```python
from build123d import *

# Parameters (mm, degrees)
EXTRUDE1_DEPTH                               = 38.1
F_3_8_CLEARANCE_HOLE1_D                      = 10.31748
TAPPED_HOLE_FOR_1_4_20_HELICOIL3_D           = 6.7564
TAPPED_HOLE_FOR_1_4_20_HELICOIL3_DEPTH       = 22.86
TAPPED_HOLE_FOR_1_4_20_HELICOIL3_CBORE_D     = 8.09498
TAPPED_HOLE_FOR_1_4_20_HELICOIL3_CBORE_DEPTH = 15.748
TAPPED_HOLE_FOR_1_4_20_HELICOIL3_TIP         = 2.029827343
TAPPED_HOLE_FOR_1_4_20_HELICOIL1_D           = 6.7564
TAPPED_HOLE_FOR_1_4_20_HELICOIL1_CBORE_D     = 8.09498
TAPPED_HOLE_FOR_1_4_20_HELICOIL1_CBORE_DEPTH = 15.748
FILLET1_R                                    = 5.08
F_3_16_0_1875_DIAMETER_HOLE1_REACH           = 70.58
F_3_16_0_1875_DIAMETER_HOLE1_BORE_R          = 2.38125
CHAMFER1_SIZE                                = 2.54


with BuildPart() as part:
    # Sketch1 → Extrude1 (new body)
    with BuildSketch(Plane.XY):
        Polygon((-73.66, 49.53), (-73.66, 68.58), (0, 68.58), (0, 0), (-38.1, 0), (-38.1, 49.53), align=None)
    extrude(amount=EXTRUDE1_DEPTH)

    # 3/8 Clearance Hole1 (through all)
    with Locations(Plane(origin=(-59.69, 68.58, 19.05), x_dir=(0, 0, 1), z_dir=(0, 1, 0))):
        with Locations((0, 0)):
            Hole(F_3_8_CLEARANCE_HOLE1_D / 2)

    # Tapped Hole for 1/4-20 Helicoil3
    with Locations(Plane(origin=(0, 59.563, 19.05), x_dir=(0, 0, 1), z_dir=(1, 0, 0))):
        with Locations((0, 0)):
            CounterBoreHole(TAPPED_HOLE_FOR_1_4_20_HELICOIL3_D / 2, TAPPED_HOLE_FOR_1_4_20_HELICOIL3_CBORE_D / 2, TAPPED_HOLE_FOR_1_4_20_HELICOIL3_CBORE_DEPTH, depth=TAPPED_HOLE_FOR_1_4_20_HELICOIL3_DEPTH)
            with Locations((0, 0, -(TAPPED_HOLE_FOR_1_4_20_HELICOIL3_DEPTH + TAPPED_HOLE_FOR_1_4_20_HELICOIL3_TIP / 2))):  # 118° drill point
                Cone(0, TAPPED_HOLE_FOR_1_4_20_HELICOIL3_D / 2, TAPPED_HOLE_FOR_1_4_20_HELICOIL3_TIP, mode=Mode.SUBTRACT)

    # Tapped Hole for 1/4-20 Helicoil1 (through all)
    with Locations(Plane(origin=(0, 14.986, 19.05), x_dir=(0, 0, 1), z_dir=(1, 0, 0))):
        with Locations((0, 0)):
            CounterBoreHole(TAPPED_HOLE_FOR_1_4_20_HELICOIL1_D / 2, TAPPED_HOLE_FOR_1_4_20_HELICOIL1_CBORE_D / 2, TAPPED_HOLE_FOR_1_4_20_HELICOIL1_CBORE_DEPTH)

    # Fillet1
    fillet1_edges = [part.edges().sort_by_distance(p)[0] for p in [
        (-38.1, 49.53, 19.05),
    ]]
    fillet(fillet1_edges, radius=FILLET1_R)

    # 3/16 (0.1875) Diameter Hole1 bore (on position points) → 3/16 (0.1875) Diameter Hole1 (cut, up to next)
    with BuildSketch(Plane(origin=(-19.05, 68.58, 19.05), x_dir=(0, 0, 1), z_dir=(0, 1, 0)), mode=Mode.PRIVATE) as f_3_16_0_1875_diameter_hole1_sk1:
        Circle(F_3_16_0_1875_DIAMETER_HOLE1_BORE_R)
    f_3_16_0_1875_diameter_hole1_tool1 = extrude(f_3_16_0_1875_diameter_hole1_sk1.sketch, amount=-F_3_16_0_1875_DIAMETER_HOLE1_REACH, mode=Mode.PRIVATE) & part.part
    add(f_3_16_0_1875_diameter_hole1_tool1.solids().sort_by_distance((-19.05, 68.58, 19.05))[0], mode=Mode.SUBTRACT)

    # Chamfer1
    chamfer1_edges = [part.edges().sort_by_distance(p)[0] for p in [
        (0, 34.29, 38.1),
        (-36.83, 68.58, 38.1),
        (-73.66, 59.055, 38.1),
        (-73.66, 59.055, 0),
        (-36.83, 68.58, 0),
        (0, 34.29, 0),
    ]]
    chamfer(chamfer1_edges, length=CHAMFER1_SIZE)


solid = part.part
```
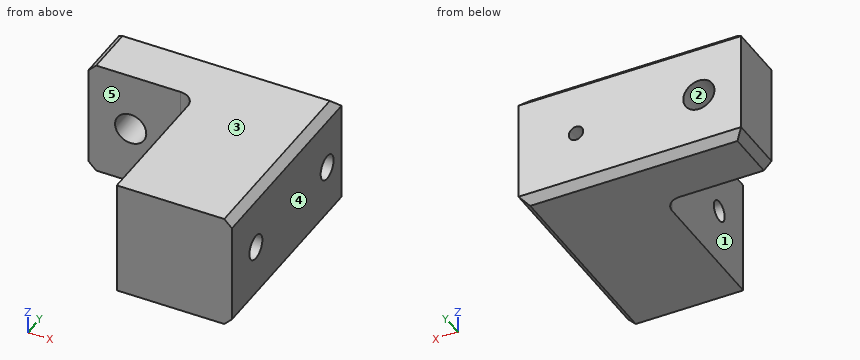
Check sheet for the modelled part. Datum: model origin and axes. Units: mm. Face numbers are marked on the shaded views. A direction names the side the tool comes from. Round coordinates to 2 decimals unless told otherwise and drop trailing zeros. Loops run counter-clockwise (first coordinate to the right, second up) from the corner with the lowest first, then second, coordinate; pieces in that order, holes last. Notation, with made-up numbers: (-39, 55.5) - (6, 55.5) arc R24 cw to (6, 65.5) - close; hole circle Ø6 at (18.25, -36.75). An arc over 180 degrees is marked (long way). Answer as a JSON object with one key per item and string values. Group by question number.
Q1. Scan lines: line 1 along X through (y, z) = (64.5, 19.05); line 2 along Y through (x, z) = (-17.5, 19.05); line 3 along Y through (x, z) = (-11.5, 16.5). Record each from-to range of solid material in increasing order. Write a range as [from, to].
Q2. Sectioned sample at C-C, the plane z = 13. Enter the section's corners in (x, y), plus the area to 3 significant figures.
Q3. Mould release check, pull along X, two halves, no side actions. Record for the marked faces 1, 2 and 3: released by +X, released by -X, zero draft, split by the parting line, or undercut.
Q4. Sectioned sample at B-B, the plane y = 51.5. Enter the section's corners in (x, z).
Q5. Sectioned sample at D-D, the plane x = -27. Enter the section's corners in (y, z).
Q6. Set-up check for the marked faces 4 and 5: record each of +Z, -Z, +X, -X, +Y, -Y from which the full face is reachable in a straight line by a thin tool's end or side.
Q7. Sectioned sample at A-A, the plane x = -59.69. Enter the section's corners in (y, z), plus the area to 3 significant figures.
Q8. Gauge pin test, flat ends, axial feed: P1, Ø4, axis at y = 59.563, z = 19.05, coming from the +X side; P2, Ø12, axis at x = -50, z = 20.5, coming from the -Y side; P3, Ø7.5, axis at y = 14.986, z = 19.05, coming from the -X side. Record the tip position at first contact, or that the pin passes through.
Solution:
{
 "1": {"line 1": "x = [-73.66, -64.85], [-54.53, -21.43], [-16.67, 0]", "line 2": "y = [0, 11.61], [18.36, 56.18]", "line 3": "y = [0, 11.84], [18.13, 56.42], [62.71, 68.58]"},
 "2": {"outline": "(-73.66, 49.53) - (-43.18, 49.53) arc R5.08 cw to (-38.1, 44.45) - (-38.1, 0) - (0, 0) - (0, 68.58) - (-73.66, 68.58) - close", "area": "3,300 mm²"},
 "3": {"face 1": "released by -X", "face 2": "undercut", "face 3": "zero draft"},
 "4": {"outline": "(-73.66, 2.54) - (-71.12, 0) - (-2.54, 0) - (0, 2.54) - (0, 35.56) - (-2.54, 38.1) - (-71.12, 38.1) - (-73.66, 35.56) - close; hole circle Ø10.32 at (-59.69, 19.05)"},
 "5": {"outline": "(0, 0) - (66.04, 0) - (68.58, 2.54) - (68.58, 35.56) - (66.04, 38.1) - (0, 38.1) - close; hole circle Ø6.76 at (14.99, 19.05)"},
 "6": {"face 4": "+Z, -Z, +X, +Y, -Y", "face 5": "+Z, -Z, -X, -Y"},
 "7": {"outline": "(49.53, 0) - (66.04, 0) - (68.58, 2.54) - (68.58, 13.89) - (49.53, 13.89) - close; (49.53, 24.21) - (68.58, 24.21) - (68.58, 35.56) - (66.04, 38.1) - (49.53, 38.1) - close", "area": "523 mm²"},
 "8": {"P1": "stops at x = -23.69", "P2": "stops at y = 49.53", "P3": "stops at x = -38.1"}
}
